The model under review builds one solid part; all positions refer to its coordinate system, in mm. Face numbers are marked on the shaded views. A direction names the side the tool comes from. Coordinates: 2 decimals unless noted, no trailing zeros. Order: outer loops, then holes, each group sorted by start corner. A loop starts at its lowest first (then second) coordinate and runs counter-clockwise, first axis right, second up.
```python
from build123d import *

# Parameters (mm, degrees)
F0_R      = 6.5
F1_DEPTH  = 6
F2_R      = 4.8
F3_DEPTH  = 7
F4_R      = 6.5
F4_R_2    = 4.8
F5_DEPTH  = 1
F6_R      = 2.5
F7_DEPTH  = 14.001
F9_R      = 4.9
F9_R_2    = 4.8
F10_DEPTH = 0.05


with BuildPart() as f1:
    # F0 (on Top) → F1 (new body)
    with BuildSketch(Plane.XY):
        Circle(F0_R)
    extrude(amount=F1_DEPTH)

    # F2 (on face) → F3 (join)
    with BuildSketch(Plane.XY.offset(6)):
        Circle(F2_R)
    extrude(amount=F3_DEPTH)

    # F4 (on face) → F5 (join)
    with BuildSketch(Plane.XY.offset(13)):
        Circle(F4_R)
        Circle(F4_R_2, mode=Mode.SUBTRACT)
        Circle(F4_R_2)
    extrude(amount=F5_DEPTH)

    # F6 (on face) → F7 (cut, through all)
    with BuildSketch(Plane.XY.offset(14)):
        Circle(F6_R)
    extrude(amount=-F7_DEPTH, mode=Mode.SUBTRACT)

    # F9 (on mid) → F10 (join, symmetric)
    with BuildSketch(Plane.XY.offset(9.5)):
        Circle(F9_R)
        Circle(F9_R_2, mode=Mode.SUBTRACT)
    extrude(amount=F10_DEPTH, both=True)


solid = f1.part
```
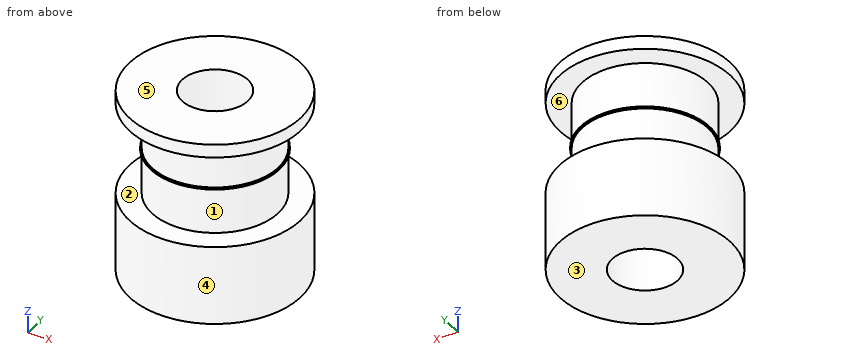
(1) Machinability: for the marked faces 5 and 6, which of the approach directions +Z, -Z, +X, -X, +Y, -Y give a long, thin tool a straight path to every point of the face, cutting with its end or side? Answer none if there is none.
A:
face 5: +Z, +X, -X, +Y, -Y
face 6: none
(2) We need section A-A, the plane x = 0. Write out the cut boundary in (y, z).
A:
outline: (-6.5, 0) - (-2.5, 0) - (-2.5, 14) - (-6.5, 14) - (-6.5, 13) - (-4.8, 13) - (-4.8, 9.55) - (-4.9, 9.55) - (-4.9, 9.45) - (-4.8, 9.45) - (-4.8, 6) - (-6.5, 6) - close; (2.5, 0) - (6.5, 0) - (6.5, 6) - (4.8, 6) - (4.8, 9.45) - (4.9, 9.45) - (4.9, 9.55) - (4.8, 9.55) - (4.8, 13) - (6.5, 13) - (6.5, 14) - (2.5, 14) - close
(3) Draft analysis for pull direction Z (two halves, no side actions). For the marked faces 1, 2, 3 and 4, state which applies: released by +Z, released by -Z, zero draft, split by the parting line, or undercut.
A:
face 1: undercut
face 2: undercut
face 3: released by -Z
face 4: zero draft
(4) For pin 1 Ø2 at (y, z) = (-2, 2) entering from -X, flat-tipped, find the tip position at first contact; note if it passes through.
A:
pin 1: stops at x = -6.42
(5) We need section C-C, the plane z = 1. Write out the cut boundary in (x, y), and give its area (3 significant figures).
A:
outline: circle Ø13 at (0, 0); hole circle Ø5 at (0, 0)
area: 113 mm2
(6) Wall thickness on probe 1 along Y at (x, z) = (0, 4.75); probe 2 along Z at (x, y) = (2.75, -4.5); probe 3 along Y at (x, z) = (0, 7): over which ranges is each line inside the solid? List them lowest first.
A:
probe 1: y = -6.5 to -2.5, 2.5 to 6.5
probe 2: z = 0 to 6, 13 to 14
probe 3: y = -4.8 to -2.5, 2.5 to 4.8
(7) We need section D-D, the plane x = 5.75. Write out the cut boundary in (y, z), and give its area (3 significant figures).
A:
outline: (-3.03, 0) - (3.03, 0) - (3.03, 6) - (-3.03, 6) - close; (-3.03, 13) - (3.03, 13) - (3.03, 14) - (-3.03, 14) - close
area: 42.4 mm2
